from build123d import *

# Parameters (mm, degrees)
SKETCH_1_R          = 2.6
SKETCH_1_R_2        = 15
SKETCH_1_W          = 20
SKETCH_1_H          = 4
EXTRUDE_1_DEPTH     = 4
SKETCH_3_W          = 20
SKETCH_3_H          = 4
EXTRUDE_2_DEPTH     = 15
SKETCH_4_R          = 1.6
CUT_EXTRUDE_1_DEPTH = 15


with BuildPart() as part:
    # 草图1 → 凸台-拉伸1 (new body)
    # profile 1 of 3: a face of its own
    with BuildSketch(Plane.XY):
        Polygon((-25, 15), (-25, 0), (-25, -21), (-5, -21), (-5, -25), (5, -25), (5, -21), (25, -21), (25, 0), (25, 15), (15, 25), (0, 25), (-15, 25), align=None)
        with Locations((0, -19)):
            Circle(SKETCH_1_R, mode=Mode.SUBTRACT)
        Circle(SKETCH_1_R_2, mode=Mode.SUBTRACT)
        with Locations((-16.592996047, 9.255943073)):
            Circle(SKETCH_1_R, mode=Mode.SUBTRACT)
        with Locations((16.309882981, 9.746164228)):
            Circle(SKETCH_1_R, mode=Mode.SUBTRACT)
    # profile 2 of 3: a face of its own
    with BuildSketch(Plane.XY):
        with Locations((15, -23)):
            Rectangle(SKETCH_1_W, SKETCH_1_H)
    # profile 3 of 3: a face of its own
    with BuildSketch(Plane.XY):
        with Locations((-15, -23)):
            Rectangle(SKETCH_1_W, SKETCH_1_H)
    extrude(amount=EXTRUDE_1_DEPTH)

    # 草图3 → 凸台-拉伸2 (add)
    with BuildSketch(Plane(origin=(0, 0, 0), x_dir=(-1, 0, 0), z_dir=(0, 0, -1))):
        with Locations((-15, -23)):
            Rectangle(SKETCH_3_W, SKETCH_3_H)
        with Locations((15, -23)):
            Rectangle(SKETCH_3_W, SKETCH_3_H)
    extrude(amount=EXTRUDE_2_DEPTH)

    # 草图4 → 切除-拉伸1 (cut)
    with BuildSketch(Plane.XZ.offset(25)):
        with Locations(Location((-15, -10, 0), (0, 0, 270))):
            Circle(SKETCH_4_R)
        with Locations(Location((15, -10, 0), (0, 0, 270))):
            Circle(SKETCH_4_R)
    extrude(amount=-CUT_EXTRUDE_1_DEPTH, mode=Mode.SUBTRACT)


solid = part.part
Verification items for the finished model (mm, model axes). A direction names the side the tool comes from. Round coordinates to 2 decimals unless told otherwise and drop trailing zeros. Order: outer loops, then holes, each group sorted by start corner. A loop starts at its lowest first (then second) coordinate and runs counter-clockwise, first axis right, second up. Notation, with made-up numbers: (33.25, 43.5) -> (48.25, 43.5) arc R16 ccw to (48.25, 74.5) -> close; hole circle Ø11 at (-18.75, -32). An arc over 180 degrees is marked (long way). Put each result on its own line as item: value.
1) Depth check by flat-ended pin: pin 1 (3.5 mm diameter, centred on x = -15, z = -10, fed in from -Y); pin 2 (7 mm diameter, centred on x = 16.31, y = 9.75, fed in from -Z); pin 3 (7.5 mm diameter, centred on x = 18.5, z = -7.5, fed in from +Y). Enter the tip coordinate at first touch or a pass-through.
Final values:
pin 1: stops at y = -25
pin 2: stops at z = 0
pin 3: stops at y = -21
2) Section check D-D (z = -5.5). Record the cut outline in (x, y), then the cut area to 3 significant figures.
Final values:
outline: (-25, -25) -> (-5, -25) -> (-5, -21) -> (-25, -21) -> close; (5, -25) -> (25, -25) -> (25, -21) -> (5, -21) -> close
area: 160 mm^2
3) Section check B-B (z = -10). Record the cut outline in (x, y), then the cut area to 3 significant figures.
Final values:
outline: (-25, -25) -> (-16.6, -25) -> (-16.6, -21) -> (-25, -21) -> close; (-13.4, -25) -> (-5, -25) -> (-5, -21) -> (-13.4, -21) -> close; (5, -25) -> (13.4, -25) -> (13.4, -21) -> (5, -21) -> close; (16.6, -25) -> (25, -25) -> (25, -21) -> (16.6, -21) -> close
area: 134 mm^2
4) Section check A-A (y = -19). Record the cut outline in (x, z).
Final values:
outline: (-25, 0) -> (-2.6, 0) -> (-2.6, 4) -> (-25, 4) -> close; (2.6, 0) -> (25, 0) -> (25, 4) -> (2.6, 4) -> close
5) Material ranges on line 1 (X direction, y = -22.5, z = -10); line 2 (Y direction, x = 7, z = -3.25); line 3 (Y direction, x = -8, z = 1.5), recorded low to high.
Final values:
line 1: x = -25 to -16.6, -13.4 to -5, 5 to 13.4, 16.6 to 25
line 2: y = -25 to -21
line 3: y = -25 to -12.69, 12.69 to 25
6) Set-up check for faces 5 (the cylindrical face through (16.08, -23.03, -8.82)), 6 (the flat face through (15, -21, -7)), 7 (the flat face through (-5, -23, -7)): record each of +Z, -Z, +X, -X, +Y, -Y from which the full face is reachable in a straight line by a thin tool's end or side.
Final values:
face 5: +Y, -Y
face 6: -Z, +X, -X, +Y
face 7: -Z, +Y, -Y
7) Section check C-C (x = 0). Record the cut outline in (y, z).
Final values:
outline: (-25, 0) -> (-21.6, 0) -> (-21.6, 4) -> (-25, 4) -> close; (-16.4, 0) -> (-15, 0) -> (-15, 4) -> (-16.4, 4) -> close; (15, 0) -> (25, 0) -> (25, 4) -> (15, 4) -> close
8) Mould release check, pull along Y, two halves, no side actions. Record for faces 1 (the flat face through (-15, -21, -7)), 2 (the flat face through (25, -9.5, 0.2)), 3 (the flat face through (6, -25, -5)), 4 (the cylindrical face through (-0.338, -16.422, 1.972)): +Y half, -Y half, draft (parallel to the pull), parting line (faces both ways), or undercut.
Final values:
face 1: +Y half
face 2: draft
face 3: -Y half
face 4: undercut
